Could you check a few things on this drawing? It's one solid part, dimensions in mm from its lowest x, y, z. A direction names the side the tool comes from. Give positions to 0.01 mm unless a question says otherwise; leave off trailing zeros. Order: outer loops, then holes, each group sorted by start corner. A loop starts at its lowest first (then second) coordinate and runs counter-clockwise, first axis right, second up.
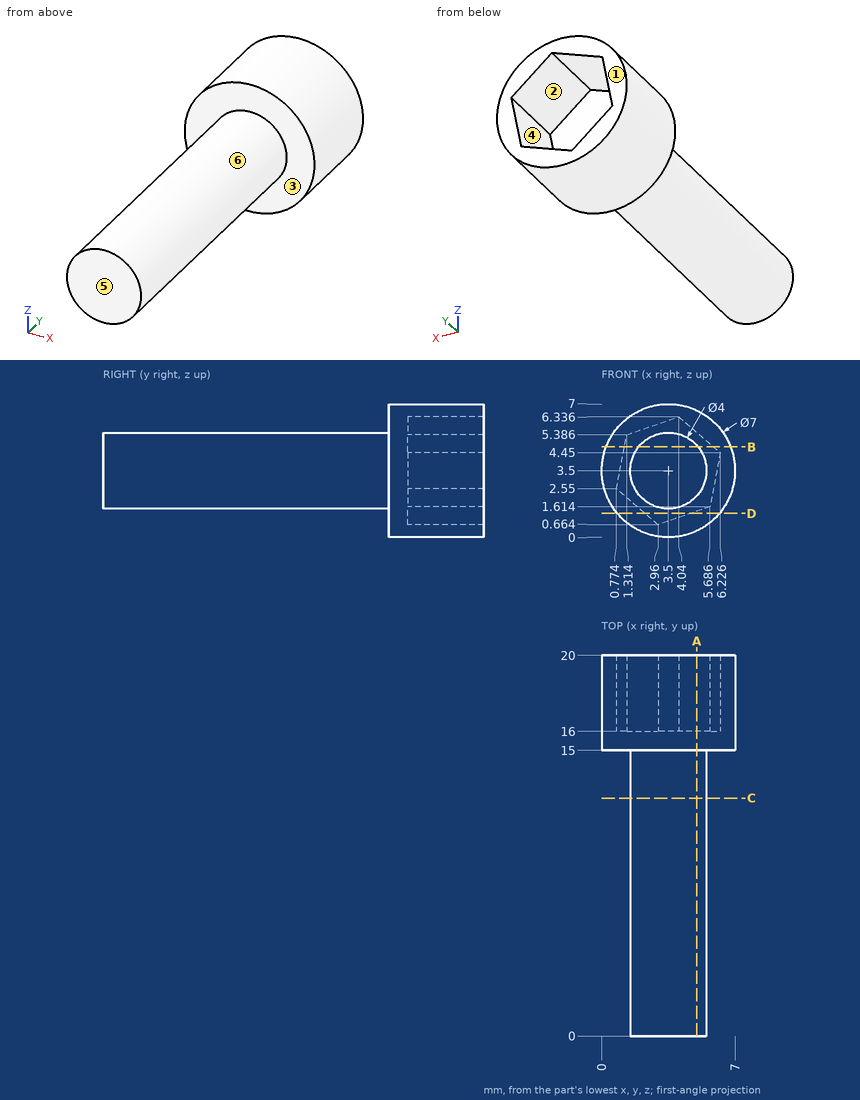
Q1. If we section it at D-D on z = 1.25: List the corners of the cut face in (x, y) for me.
Filled sheet:
outline: (0.82, 15) - (6.18, 15) - (6.18, 20) - (4.64, 20) - (4.64, 16) - (2.28, 16) - (2.28, 20) - (0.82, 20) - close
Q2. I'm going to push flat-ended pins straight in: P1, Ø2, axis at y = 10, z = 6, coming from the +X side; P2, Ø4, axis at x = 3.5, y = 9.5, coming from the -Z side; P3, Ø3, axis at x = 1.5, y = 14, coming from the -Z side. Where does each tip first touch, or does it pass through?
Filled sheet:
P1: stops at x = 4.82
P2: stops at z = 1.5
P3: stops at z = 0.11
Q3. I need wall thicknesses on L1, parallel to Y at x = 2.5, z = 4.25; L2, parallel to Y at x = 3.25, z = 0.5; L3, parallel to X at y = 18, z = 3.5 (1 decimal). Which ranges of each line are inside material? Lowest first, please.
Filled sheet:
L1: y = 0 to 16
L2: y = 15 to 20
L3: x = 0 to 1, 6 to 7
Q4. If we section it at C-C on y = 12.5: List the corners of the cut face in (x, z) for me.
Filled sheet:
outline: circle Ø4 at (3.5, 3.5)
Q5. If we section it at B-B on z = 4.75: List the corners of the cut face in (x, y) for me.
Filled sheet:
outline: (0.23, 15) - (1.94, 15) - (1.94, 0) - (5.06, 0) - (5.06, 15) - (6.77, 15) - (6.77, 20) - (5.88, 20) - (5.88, 16) - (1.19, 16) - (1.19, 20) - (0.23, 20) - close
Q6. If we section it at A-A on x = 5: List the corners of the cut face in (y, z) for me (1 decimal).
Filled sheet:
outline: (0, 2.2) - (15, 2.2) - (15, 0.3) - (20, 0.3) - (20, 1.4) - (16, 1.4) - (16, 5.5) - (20, 5.5) - (20, 6.7) - (15, 6.7) - (15, 4.8) - (0, 4.8) - close
Q7. Thinking about a two-plate mould opening in Z: for the marked faces 4, 5 and 6, which applies, released by +Z, released by -Z, zero draft, split by the parting line, or undercut?
Filled sheet:
face 4: undercut
face 5: zero draft
face 6: split by the parting line
Q8. For the marked faces 1, 2 and 3, which set-ups out of +Z, -Z, +X, -X, +Y, -Y let a thin tool reach every point of the face, with its end or its side?
Filled sheet:
face 1: +Z, -Z, +X, -X, +Y
face 2: +Y
face 3: -Y
